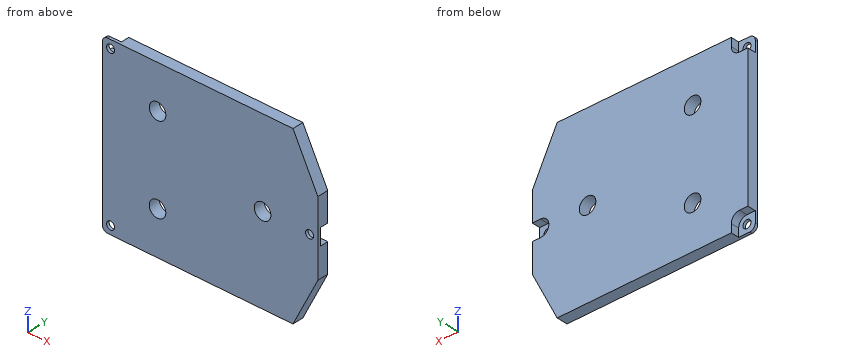
from build123d import *

# Parameters (mm, degrees)
SALIENTE_EXTRUIR1_DEPTH = 4
CROQUIS2_R              = 1.45
CORTAR_EXTRUIR1_DEPTH   = 4
REDONDEO1_R             = 2
CORTAR_EXTRUIR2_DEPTH   = 3
CROQUIS4_R              = 3
CORTAR_EXTRUIR3_DEPTH   = 10


with BuildPart() as part:
    # Croquis1 → Saliente-Extruir1 (new body)
    with BuildSketch(Plane(origin=(0, 0, 0), x_dir=(1, 0, 0), z_dir=(0, 1, 0))):
        Polygon((63, 0), (69, 0), (78, 18), (78, 45), (69, 63), (63, 63), (0, 63), (0, 0), align=None)
    extrude(amount=SALIENTE_EXTRUIR1_DEPTH)

    # Croquis2 → Cortar-Extruir1 (cut)
    with BuildSketch(Plane(origin=(0, 4, 0), x_dir=(1, 0, 0), z_dir=(0, 1, 0))):
        with Locations(Location((3, 3, 0), (0, 0, 270))):
            Circle(CROQUIS2_R)
        with Locations(Location((3, 60, 0), (0, 0, 270))):
            Circle(CROQUIS2_R)
        with Locations(Location((75, 31.5, 0), (0, 0, 270))):
            Circle(CROQUIS2_R)
    extrude(amount=-CORTAR_EXTRUIR1_DEPTH, mode=Mode.SUBTRACT)

    # Redondeo1
    redondeo1_edges = [part.edges().sort_by_distance(p)[0] for p in [
        (0, 2, -63),
        (0, 2, 0),
    ]]
    fillet(redondeo1_edges, radius=REDONDEO1_R)

    # Croquis3 → Cortar-Extruir2 (cut)
    with BuildSketch(Plane(origin=(0, 4, 0), x_dir=(1, 0, 0), z_dir=(0, 1, 0))):
        with BuildLine():
            Line((6, 3), (6, 0))
            Line((6, 0), (0, 0))
            Line((0, 0), (0, 3))
            Line((0, 3), (0, 6))
            Line((0, 6), (3, 6))
            ThreePointArc((3, 6), (5.121320344, 5.121320344), (6, 3))
        make_face()
        with BuildLine():
            Line((3, 57), (0, 57))
            Line((0, 57), (0, 63))
            Line((0, 63), (6, 63))
            Line((6, 63), (6, 60))
            ThreePointArc((6, 60), (5.121320344, 57.878679656), (3, 57))
        make_face()
        with BuildLine():
            Line((75, 28.5), (78, 28.5))
            Line((78, 28.5), (78, 34.5))
            Line((78, 34.5), (75, 34.5))
            ThreePointArc((75, 34.5), (72, 31.5), (75, 28.5))
        make_face()
    extrude(amount=-CORTAR_EXTRUIR2_DEPTH, mode=Mode.SUBTRACT)

    # Croquis4 → Cortar-Extruir3 (cut)
    with BuildSketch(Plane(origin=(0, 4, 0), x_dir=(1, 0, 0), z_dir=(0, 1, 0))):
        with Locations(Location((20, 47.25, 0), (0, 0, 270))):
            Circle(CROQUIS4_R)
        with Locations(Location((20, 15.75, 0), (0, 0, 270))):
            Circle(CROQUIS4_R)
        with Locations(Location((58, 31.5, 0), (0, 0, 270))):
            Circle(CROQUIS4_R)
    extrude(amount=-CORTAR_EXTRUIR3_DEPTH, mode=Mode.SUBTRACT)


solid = part.part
Design review of the part built by this model. Coordinates are the model's own, in mm. Give positions to 0.01 mm unless a question says otherwise; leave off trailing zeros. Loops run counter-clockwise (first coordinate to the right, second up) from the corner with the lowest first, then second, coordinate; pieces in that order, holes last. Notation, with made-up numbers: (46.5, -12.5) -> (52.5, -12.5) arc R17 ccw to (52.5, 9.5) -> close; hole circle Ø5 at (9.25, 21.25). An arc over 180 degrees is marked (long way). One line per question, with ' | ' between items. Start each with the question number.
(1) We need section C-C (z = -47.25). State the section outline as (x, y) points (3 decimals), and give its area (4 significant figures).
(2) For line 1 (X direction, y = 0.7, z = -31.5); line 2 (Z direction, x = 19.5, y = 0.4); line 3 (Z direction, x = 74, y = 3.85), list the stretches that pass through material, from the lowest coordinate up.
(3) We need section A-A (x = 20). State the section outline as (y, z) points.
(4) Insertion check: P1, Ø1.8, axis at x = 4, z = -59, coming from the +Y side; P2, Ø5.5, axis at x = 20, z = -15.75, coming from the +Y side; P3, Ø0.9, axis at x = 76, y = 3, coming from the -Z side; P4, Ø1.5, axis at y = 2, z = -62, coming from the -X side. Each pin has a flat end and moves straight along its axis. Give the tip position at first contact, or say it passes through.
(5) We need section B-B (y = 2.65). State the section outline as (x, z) points.
(6) We need section D-D (z = -7.5). State the section outline as (x, y) points, and give its area (3 significant figures).
The answers:
1) outline: (0, 0) -> (17, 0) -> (17, 4) -> (0, 4) -> close; (23, 0) -> (76.875, 0) -> (76.875, 4) -> (23, 4) -> close | area: 283.5 mm^2
2) line 1: x = 0 to 55, 61 to 73.55, 76.45 to 78 | line 2: z = -63 to -50.21, -44.29 to -18.71, -12.79 to 0 | line 3: z = -53 to -34.33, -28.67 to -10
3) outline: (0, -63) -> (4, -63) -> (4, -50.25) -> (0, -50.25) -> close; (0, -44.25) -> (4, -44.25) -> (4, -18.75) -> (0, -18.75) -> close; (0, -12.75) -> (4, -12.75) -> (4, 0) -> (0, 0) -> close
4) P1: stops at y = 1 | P2: passes through | P3: stops at z = -49.9 | P4: stops at x = 6
5) outline: (0, -57) -> (3, -57) arc R3 cw to (6, -60) -> (6, -63) -> (69, -63) -> (78, -45) -> (78, -34.5) -> (75, -34.5) arc R3 cw to (75, -28.5) -> (78, -28.5) -> (78, -18) -> (69, 0) -> (6, 0) -> (6, -3) arc R3 cw to (3, -6) -> (0, -6) -> close; hole circle Ø6 at (20, -47.25); hole circle Ø6 at (20, -15.75); hole circle Ø6 at (58, -31.5)
6) outline: (0, 0) -> (72.75, 0) -> (72.75, 4) -> (0, 4) -> close | area: 291 mm^2
